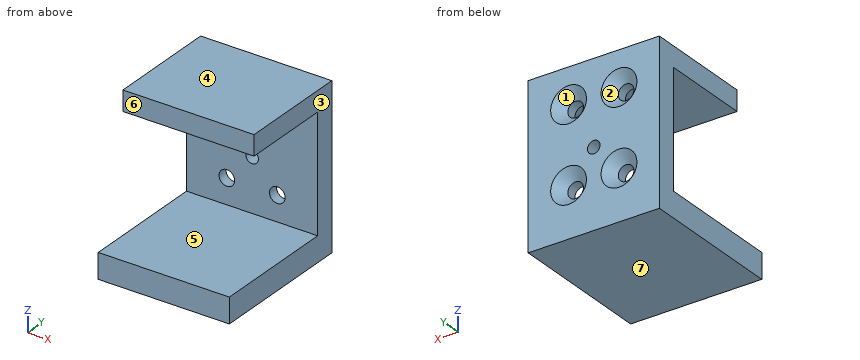
Autodesk Inventor part; units mm, degrees
ref_plane "YZ Plane" through (0, 0, 0) normal (1, 0, 0) x (0, 1, 0)
ref_plane "XZ Plane" through (0, 0, 0) normal (0, 1, 0) x (-1, 0, 0)
ref_plane "XY Plane" through (0, 0, 0) normal (0, 0, 1) x (1, 0, 0)
sketch "Sketch1" plane through (0, 0, 0) normal (0, 1, 0) x (-1, 0, 0)
  line L0 (13.2828, -12.6642) -> (-12.7172, -12.6642)
  line L1 (-12.7172, -12.6642) -> (-12.7172, 17.3358)
  line L2 (-12.7172, 17.3358) -> (13.2828, 17.3358)
  line L3 (13.2828, 17.3358) -> (13.2828, -12.6642)
  point P0 (0, 0)
  dimension "d0" = 26
  dimension "d1" = 30
extrude "Extrusion1" add sketch "Sketch1" along normal blind 4
sketch "Sketch2" plane through (0, 4, 0) normal (0, 1, 0) x (1, 0, 0)
  circle A0 centre (-5.2828, 2.6642) radius 1.55
  circle A1 centre (4.7172, 2.6642) radius 1.55
  circle A2 centre (-5.2828, -12.3358) radius 1.55
  circle A3 centre (4.7172, -12.3358) radius 1.55
  line L0 (-13.2828, -17.3358) -> (12.7172, -17.3358)
  line L1 (-13.2828, 12.6642) -> (-13.2828, -17.3358)
  point P0 (0, 0)
  dimension "d4" = 3.1
  dimension "d5" = 3.1
  dimension "d6" = 3.1
  dimension "d7" = 3.1
  dimension "d8" = 10
  dimension "d9" = 10
  dimension "d10" = 15
  dimension "d11" = 15
  dimension "d12" = 5
  dimension "d13" = 5
  dimension "d14" = 8
  dimension "d15" = 8
extrude "Extrusion2" cut sketch "Sketch2" against normal through all
sketch "Sketch3" plane through (0, 0, 0) normal (0, -1, 0) x (1, 0, 0)
  point P0 (0, 0)
sketch "Sketch4" plane through (-13.2828, 0, -12.6642) normal (-1, 0, 0) x (0, 0, 1)
  line L0 (30, 4) -> (0, 4)
  line L1 (28, 4) -> (32, 4)
  line L2 (32, 4) -> (32, -18)
  line L3 (32, -18) -> (28, -18)
  line L4 (28, -18) -> (28, 4)
  line L5 (30, 0) -> (30, 4)
  point P0 (12.6642, 0)
  dimension "d18" = 2
  dimension "d19" = 4
  dimension "d20" = 22
extrude "Extrusion3" add sketch "Sketch4" against normal up to surface (26 mm away)
chamfer "Chamfer1" distance 2 angle 45 4 edges at (-6.8328, 4, 12.3358) (3.1672, 4, 12.3358) (-6.8328, 4, -2.6642) (3.1672, 4, -2.6642)
sketch "Sketch5" plane through (0, 4, 0) normal (0, 1, 0) x (1, 0, 0)
  circle A0 centre (-0.2828, -2.8358) radius 1.25
  line L0 (12.7172, 12.6642) -> (-13.2828, 12.6642)
  line L1 (-13.2828, 12.6642) -> (-13.2828, -19.3358)
  point P0 (0, 0)
  dimension "d26" = 2.5
  dimension "d27" = 15.5
  dimension "d28" = 13
extrude "Extrusion4" cut sketch "Sketch5" against normal through all
sketch "Sketch6" plane through (0, 0, 0) normal (0, -1, 0) x (1, 0, 0)
  line L0 (12.7172, -12.6642) -> (-13.2828, -12.6642)
  line L1 (-13.2828, -12.6642) -> (12.7172, -12.6642)
  line L2 (12.7172, -12.6642) -> (12.7172, -7.6642)
  line L3 (12.7172, -7.6642) -> (-13.2828, -7.6642)
  line L4 (-13.2828, -7.6642) -> (-13.2828, -12.6642)
  point P0 (0, 0)
  dimension "d31" = 5
extrude "Extrusion5" add sketch "Sketch6" along normal blind 25
properties part number "grantry_holder_R"
The listing builds one solid part. Answer for the finished solid, in the listing's coordinates (mm). Face numbers are marked on the shaded views. A direction names the side the tool comes from. Round coordinates to 2 decimals unless told otherwise and drop trailing zeros. Loops run counter-clockwise (first coordinate to the right, second up) from the corner with the lowest first, then second, coordinate; pieces in that order, holes last.
Q1. Find the intervals of material crossed by line 1 (Z direction, x = -6, y = -16); line 2 (Y direction, x = -8, z = 16); line 3 (Y direction, x = 7.75, z = -5.5), in increasing order.
Q2. Which of the six approach directions +Z, -Z, +X, -X, +Y, -Y give full straight-line access (tool end or side, diameter ignored) to the marked faces 5, 6 and 7?
Q3. Section B-B, the plane x = -11 is taken. Determine the outline of the cut face in (y, z), then the cut area to 3 significant figures.
Q4. Section D-D, the plane x = 0.5 is taken. Determine the outline of the cut face in (y, z).
Q5. For a pull along X with two mould halves and no side action, classify the marked faces 1, 2, 3 and 4 as released by +X, released by -X, zero draft, split by the parting line, or undercut.
Q6. Section A-A, the plane y = -6 is taken. Determine the outline of the cut face in (x, z), then the cut area to 3 significant figures.
Q7. Section C-C, the plane z = 2 is taken. Determine the outline of the cut face in (x, y), then the cut area to 3 significant figures.
Q8. Given pin 1 Ø3.5 at (x, z) = (-5.28, 12.34) entering from +Y; pin 2 Ø3 at (x, z) = (8, 2) entering from -Y; pin 3 Ø4.5 at (x, z) = (0.5, 17) entering from -Y; pin 4 Ø12 at (y, z) = (-21, 15) entering from +X, each flat-ended and moving along its own axis, determine where each tip first touches the part or whether it passes through.
Completed:
1. line 1: z = -12.66 to -7.66, 15.34 to 19.34
1. line 2: y = -18 to 4
1. line 3: y = 0 to 4
2. face 5: +X, -X, -Y
2. face 6: +Z, +X, -X, -Y
2. face 7: -Z, +X, -X, +Y, -Y
3. outline: (-25, -12.66) - (4, -12.66) - (4, 19.34) - (-18, 19.34) - (-18, 15.34) - (0, 15.34) - (0, -7.66) - (-25, -7.66) - close
3. area: 325 mm2
4. outline: (-25, -12.66) - (4, -12.66) - (4, 1.86) - (0, 1.86) - (0, -7.66) - (-25, -7.66) - close; (-18, 15.34) - (0, 15.34) - (0, 3.81) - (4, 3.81) - (4, 19.34) - (-18, 19.34) - close
5. face 1: undercut
5. face 2: undercut
5. face 3: released by +X
5. face 4: zero draft
6. outline: (-13.28, -12.66) - (12.72, -12.66) - (12.72, -7.66) - (-13.28, -7.66) - close; (-13.28, 15.34) - (12.72, 15.34) - (12.72, 19.34) - (-13.28, 19.34) - close
6. area: 234 mm2
7. outline: (-13.28, 0) - (-1.21, 0) - (-1.21, 4) - (-13.28, 4) - close; (0.65, 0) - (12.72, 0) - (12.72, 4) - (0.65, 4) - close
7. area: 96.6 mm2
8. pin 1: stops at y = 2.21
8. pin 2: stops at y = 0
8. pin 3: stops at y = -18
8. pin 4: stops at x = 12.72
